Study the drawing (mm; zero at the part's minimum x, y, z) and answer. A direction names the side the tool comes from. Coordinates: 2 decimals unless noted, no trailing zeros. Order: outer loops, then holes, each group sorted by start corner. A loop starts at its lowest first (then second) coordinate and runs counter-clockwise, first axis right, second up. Notation, with made-up numbers: (-40, 48.5) -> (-5, 48.5) arc R32 cw to (-5, 79.5) -> close; hole circle Ø4 at (-38.75, 36). An arc over 180 degrees is marked (long way). Answer as CSV lines item,"result". Start each with the question number.
Item 1: Each of these flat-tipped pins is pushed along its axis until it touches: pin 1 Ø2 at (x, z) = (10.5, 35.75) entering from +Y; pin 2 Ø4.5 at (x, z) = (8.5, 21) entering from -Y; pin 3 Ø4 at (x, y) = (3, 7.5) entering from -Z. Where does it stop, or does it pass through?
Item 2: For a pull along Z with two mould halves and no side action, classify the marked faces 3, 4 and 5 as pulls with the +Z half, pulls with the -Z half, needs draft (parallel to the pull), parting line crosses it, or undercut.
Item 3: Straight lines are drawn through the part: L1, parallel to Z at x = 10.5, y = 7.5; L2, parallel to Z at x = 7.75, y = 5.75; L3, parallel to Z at x = 3.75, y = 6. For each, find the intervals that lie inside material, in ascending order.
Item 4: Section A-A (y = 9.25) is taken. Write down the section's boundary in (x, z).
Item 5: Section C-C (z = 4.25) is taken. Write down the section's boundary in (x, y).
Item 6: Section D-D (x = 5.5) is taken. Write down the section's boundary in (y, z), then the cut area to 4 significant figures.
Item 7: Section B-B (x = 10.5) is taken. Write down the section's boundary in (y, z).
Item 8: Which of the six approach directions +Z, -Z, +X, -X, +Y, -Y give full straight-line access (tool end or side, diameter ignored) to the marked faces 1 and 2?
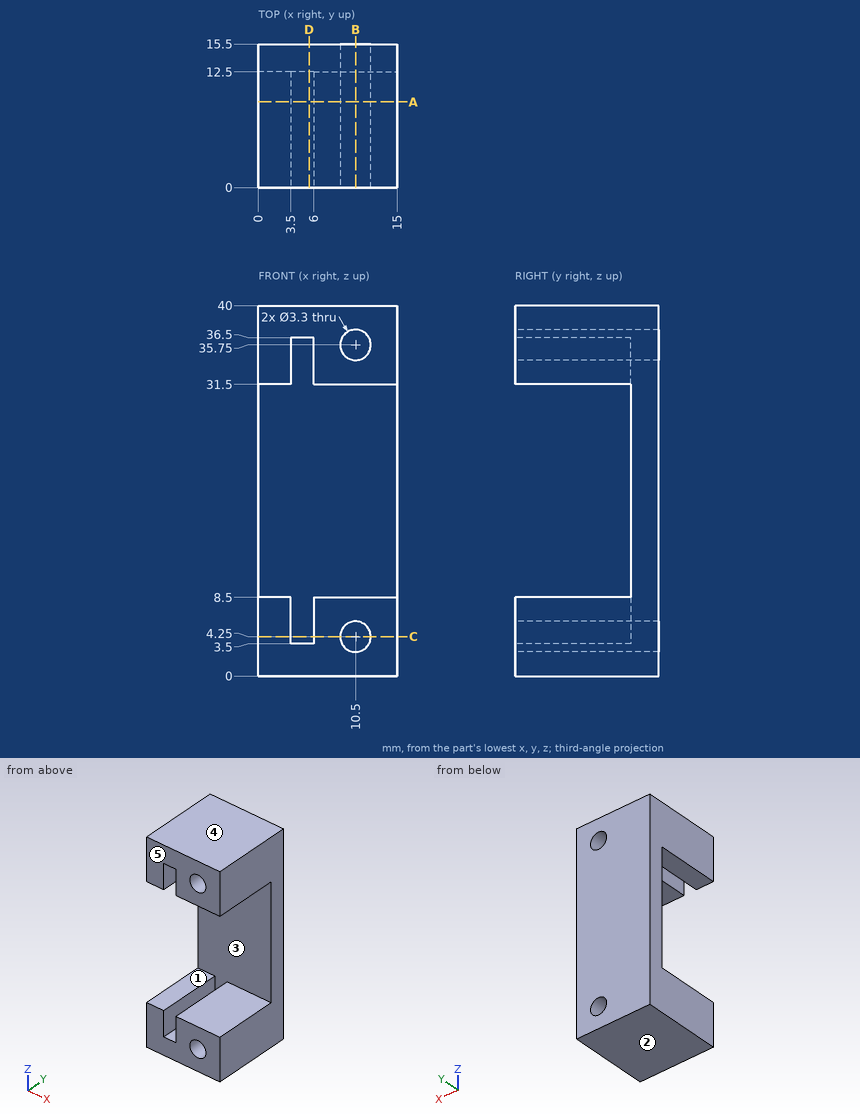
Checked values:
1,pin 1,"passes through"
1,pin 2,"stops at y = 12.5"
1,pin 3,"stops at z = 0"
2,face 3,"undercut"
2,face 4,"pulls with the +Z half"
2,face 5,"needs draft"
3,L1,"z = 0 to 2.6, 5.9 to 8.5, 31.5 to 34.1, 37.4 to 40"
3,L2,"z = 0 to 8.5, 31.5 to 40"
3,L3,"z = 0 to 3.5, 36.5 to 40"
4,outline,"(0, 0) -> (15, 0) -> (15, 8.5) -> (6, 8.5) -> (6, 3.5) -> (3.5, 3.5) -> (3.5, 8.5) -> (0, 8.5) -> close; (0, 31.5) -> (3.5, 31.5) -> (3.5, 36.5) -> (6, 36.5) -> (6, 31.5) -> (15, 31.5) -> (15, 40) -> (0, 40) -> close; hole circle Ø3.3 at (10.5, 4.25); hole circle Ø3.3 at (10.5, 35.75)"
5,outline,"(0, 0) -> (3.5, 0) -> (3.5, 12.5) -> (6, 12.5) -> (6, 0) -> (8.85, 0) -> (8.85, 15.5) -> (0, 15.5) -> close; (12.15, 0) -> (15, 0) -> (15, 15.5) -> (12.15, 15.5) -> close"
6,outline,"(0, 0) -> (15.5, 0) -> (15.5, 40) -> (0, 40) -> (0, 36.5) -> (12.5, 36.5) -> (12.5, 3.5) -> (0, 3.5) -> close"
6,area,"207.5 mm^2"
7,outline,"(0, 0) -> (15.5, 0) -> (15.5, 2.6) -> (0, 2.6) -> close; (0, 5.9) -> (15.5, 5.9) -> (15.5, 34.1) -> (0, 34.1) -> (0, 31.5) -> (12.5, 31.5) -> (12.5, 8.5) -> (0, 8.5) -> close; (0, 37.4) -> (15.5, 37.4) -> (15.5, 40) -> (0, 40) -> close"
8,face 1,"+X, -X, -Y"
8,face 2,"-Z, +X, -X, +Y, -Y"
